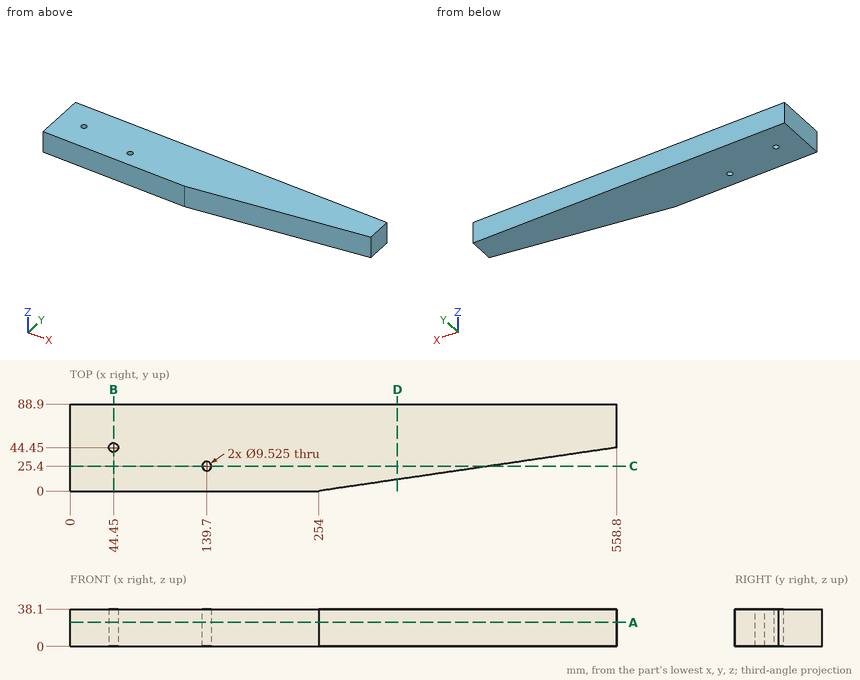
The figure shows three views and two pictorial views of one solid part (mm, origin at its lowest corner). Answer the questions. Round coordinates to 2 decimals unless told otherwise and drop trailing zeros. Order: outer loops, then holes, each group sorted by start corner. A loop starts at its lowest first (then second) coordinate and runs counter-clockwise, first axis right, second up. Notation, with made-up numbers: (0.5, 40.5) - (35.5, 40.5) arc R13 cw to (35.5, 62.5) - close; hole circle Ø1 at (3, 12.25). An arc over 180 degrees is marked (long way). Write item = value, one per line. Start each with the question number.
1) Section D-D, the plane x = 334.5 is taken. Write down the section's boundary in (y, z).
2) Section B-B, the plane x = 44.45 is taken. Write down the section's boundary in (y, z), plus the area to 3 significant figures.
3) Section C-C, the plane y = 25.4 is taken. Write down the section's boundary in (x, z), plus the area to 3 significant figures.
4) Section A-A, the plane z = 24.5 is taken. Count the separate pieces of the cut face and the enclosed holes in it, plus the area to 3 significant figures.
5) Given pin 1 (10 mm diameter, centred on x = 203.5, y = 70.5, fed in from -Z), flat-ended and moving along its own axis, determine where the tip first touches the part or whether it passes through.
6) Straight lines are drawn through the part: L1, parallel to Y at x = 44.45, z = 13.5; L2, parallel to Y at x = 139, z = 9; L3, parallel to Y at x = 335.5, z = 18.5. For each, find the intervals that lie inside material, in ascending order.
Results list:
q1.outline = (11.74, 0) - (88.9, 0) - (88.9, 38.1) - (11.74, 38.1) - close
q2.outline = (0, 0) - (39.69, 0) - (39.69, 38.1) - (0, 38.1) - close; (49.21, 0) - (88.9, 0) - (88.9, 38.1) - (49.21, 38.1) - close
q2.area = 3,020 mm^2
q3.outline = (0, 0) - (134.94, 0) - (134.94, 38.1) - (0, 38.1) - close; (144.46, 0) - (428.17, 0) - (428.17, 38.1) - (144.46, 38.1) - close
q3.area = 16,000 mm^2
q4.separate_pieces = 1
q4.enclosed_holes = 2
q4.area = 42,800 mm^2
q5.pin_1 = 0
q6.L1 = 0 to 39.69, 49.21 to 88.9
q6.L2 = 0 to 20.69, 30.11 to 88.9
q6.L3 = 11.89 to 88.9
